The model under review builds one solid part; all positions refer to its coordinate system, in mm. A direction names the side the tool comes from. Coordinates: 2 decimals unless noted, no trailing zeros. Order: outer loops, then holes, each group sorted by start corner. A loop starts at its lowest first (then second) coordinate and runs counter-clockwise, first axis right, second up. Notation, with made-up numbers: (33.25, 2.25) -> (83.25, 2.25) arc R8 cw to (83.25, 8.25) -> close; hole circle Ø10 at (-36, 82.5). An arc over 180 degrees is marked (long way). Use CSV: the item, a comma, the result in double quotes. Start each with the question number.
```python
from build123d import *

# Parameters (mm, degrees)
DODANIE_WYCI_GNI_CIE3_DEPTH = 10
SZKIC4_W                    = 6
SZKIC4_H                    = 24.913855362
WYTNIJ_WYCI_GNI_CIE2_DEPTH  = 22
OTW_R_POD_RUB_M21_D         = 2.6


with BuildPart() as part:
    # Szkic3 → Dodanie-wyciągnięcie3 (new body)
    with BuildSketch(Plane.XY):
        with BuildLine():
            Line((0, -10), (0, 10))
            Line((0, 10), (-3, 10))
            Line((-3, 10), (-15.604135503, 2.585802645))
            ThreePointArc((-15.604135503, 2.585802645), (-17.083075123, 0), (-15.604135503, -2.585802645))
            Line((-15.604135503, -2.585802645), (-3, -10))
            Line((-3, -10), (0, -10))
        make_face()
    extrude(amount=DODANIE_WYCI_GNI_CIE3_DEPTH)

    # Szkic4 → Wytnij-wyciągnięcie2 (cut)
    with BuildSketch(Plane(origin=(-25, 0, 0), x_dir=(0, 0, -1), z_dir=(1, 0, 0))):
        with Locations((-5, 0)):
            Rectangle(SZKIC4_W, SZKIC4_H)
    extrude(amount=WYTNIJ_WYCI_GNI_CIE2_DEPTH, mode=Mode.SUBTRACT)

    # Otwór pod śrubę M21 (through all)
    with Locations(Plane.XY.offset(10)):
        with Locations((-9, 0)):
            Hole(OTW_R_POD_RUB_M21_D / 2)


solid = part.part
```
Q1. Draft analysis for pull direction Z (two halves, no side actions). For faces 1 (the cylindrical face through (-17.083, 0.044, 8.986)), 2 (the flat face through (-7, 0, 10)), 3 (the flat face through (-7, 0, 8)), state which applies: +Z half, -Z half, draft (parallel to the pull), parting line (faces both ways), or undercut.
Q2. Add section A-A, the plane y = 0. State the section outline as (x, z) points, then the cut area to 3 significant figures.
Q3. Add section D-D, the plane x = -9. State the section outline as (y, z) points.
Q4. Clearance check with flat-ended pins moving along their axes: pin 1 Ø2 at (x, z) = (-11, 6) entering from +Y; pin 2 Ø2 at (y, z) = (-4.5, 2.5) entering from -X. State where each tip first meets the part, or that it passes through.
Q5. Add section C-C, the plane y = -7.5. State the section outline as (x, z) points.
Q6. To check wall thickness, follow probe 1 along Z at (x, y) = (-4, 7.75); probe 2 along X at (y, z) = (7.5, 4.75); probe 3 along Y at (x, z) = (-9, 9.25). State the ranges of each line that lie inside material, in increasing order.
Q7. For faces 4 (the flat face through (-3, 0, 5)), 5 (the flat face through (-2, -10, 5)), list the 3-axis set-ups (+Z, -Z, +X, -X, +Y, -Y) from which the entire face can be reached by the end or side of a thin tool; tool diameter is ignored.
Q8. Add section B-B, the plane x = -5.25. State the section outline as (y, z) points, then the cut area to 3 significant figures.
Answer block:
1,face 1,"draft"
1,face 2,"+Z half"
1,face 3,"undercut"
2,outline,"(-17.08, 0) -> (-10.3, 0) -> (-10.3, 2) -> (-17.08, 2) -> close; (-17.08, 8) -> (-10.3, 8) -> (-10.3, 10) -> (-17.08, 10) -> close; (-7.7, 0) -> (0, 0) -> (0, 10) -> (-7.7, 10) -> (-7.7, 8) -> (-3, 8) -> (-3, 2) -> (-7.7, 2) -> close"
2,area,"75.9 mm²"
3,outline,"(-6.47, 0) -> (-1.3, 0) -> (-1.3, 2) -> (-6.47, 2) -> close; (-6.47, 8) -> (-1.3, 8) -> (-1.3, 10) -> (-6.47, 10) -> close; (1.3, 0) -> (6.47, 0) -> (6.47, 2) -> (1.3, 2) -> close; (1.3, 8) -> (6.47, 8) -> (6.47, 10) -> (1.3, 10) -> close"
4,pin 1,"passes through"
4,pin 2,"stops at x = -13.82"
5,outline,"(-7.25, 0) -> (0, 0) -> (0, 10) -> (-7.25, 10) -> (-7.25, 8) -> (-3, 8) -> (-3, 2) -> (-7.25, 2) -> close"
6,probe 1,"z = 0 to 2, 8 to 10"
6,probe 2,"x = -3 to 0"
6,probe 3,"y = -6.47 to -1.3, 1.3 to 6.47"
7,face 4,"-X, +Y, -Y"
7,face 5,"+Z, -Z, +X, -X, -Y"
8,outline,"(-8.68, 0) -> (8.68, 0) -> (8.68, 2) -> (-8.68, 2) -> close; (-8.68, 8) -> (8.68, 8) -> (8.68, 10) -> (-8.68, 10) -> close"
8,area,"69.4 mm²"
